from build123d import *

# Parameters (mm, degrees)
SKETCH_1_W          = 31.500863908
SKETCH_1_H          = 82
SKETCH_1_R          = 10.417524335
SKETCH_1_R_2        = 1.56
EXTRUDE_1_DEPTH     = 4
SKETCH_3_W          = 31.500863908
SKETCH_3_H          = 3
EXTRUDE_2_DEPTH     = 35
SKETCH_6_R          = 1.5
CUT_EXTRUDE_1_DEPTH = 4


with BuildPart() as part:
    # 草图1 → 凸台-拉伸1 (new body)
    with BuildSketch(Plane.XY):
        with Locations((0, 14.377078694)):
            Rectangle(SKETCH_1_W, SKETCH_1_H)
        with Locations((0, -6.708333333)):
            Circle(SKETCH_1_R, mode=Mode.SUBTRACT)
        with Locations((0, -20.208333333)):
            Circle(SKETCH_1_R_2, mode=Mode.SUBTRACT)
        with BuildLine():
            Line((8.85, 15.791666667), (-8.85, 15.791666667))
            ThreePointArc((-8.85, 15.791666667), (-10.35, 14.291666667), (-8.85, 12.791666667))
            Line((-8.85, 12.791666667), (8.85, 12.791666667))
            ThreePointArc((8.85, 12.791666667), (10.35, 14.291666667), (8.85, 15.791666667))
        make_face(mode=Mode.SUBTRACT)
    extrude(amount=EXTRUDE_1_DEPTH)

    # 草图3 → 凸台-拉伸2 (add)
    with BuildSketch(Plane(origin=(0, 0, 0), x_dir=(-1, 0, 0), z_dir=(0, 0, -1))):
        with Locations((0, 53.877078694)):
            Rectangle(SKETCH_3_W, SKETCH_3_H)
    extrude(amount=EXTRUDE_2_DEPTH)

    # 草图6 → 切除-拉伸1 (cut, through all)
    with BuildSketch(Plane.XZ.offset(-52.377078694)):
        with Locations((-8.166436246, -9.151254402)):
            Circle(SKETCH_6_R)
        with Locations((8.166436246, -9.151254402)):
            Circle(SKETCH_6_R)
        with Locations((8.166436246, -25.848745598)):
            Circle(SKETCH_6_R)
        with Locations((-8.166436246, -25.848745598)):
            Circle(SKETCH_6_R)
    extrude(amount=-CUT_EXTRUDE_1_DEPTH, mode=Mode.SUBTRACT)


solid = part.part
The model under review builds one solid part; all positions refer to its coordinate system, in mm. A direction names the side the tool comes from. Coordinates: 2 decimals unless noted, no trailing zeros. Write each loop counter-clockwise with the first axis right and the second up, starting at its lowest first coordinate (ties: lowest second). Pieces come first, ordered by that corner, then holes. Notation, with made-up numbers: (-10, 58.5) - (-2, 58.5) arc R36 ccw to (-2, 93.5) - close; hole circle Ø9 at (35.25, 71). An arc over 180 degrees is marked (long way). Answer as CSV lines item,"result".
(1) We need section D-D (x = 12). Give the boundary of the cut face in (y, z).
Data:
outline,"(-26.62, 0) - (52.38, 0) - (52.38, -35) - (55.38, -35) - (55.38, 4) - (-26.62, 4) - close"
(2) Tool access review of faces 1 (the flat face through (0, 52.377, -17)), 2 (the cylindrical face through (10.35, 14.26, 1.97)), 3 (the flat face through (-15.75, 20.3, 0.5)): name each direction out of +Z, -Z, +X, -X, +Y, -Y from which nothing blocks a thin tool from reaching the whole face with its end or side.
Data:
face 1,"-Z, +X, -X, -Y"
face 2,"+Z, -Z"
face 3,"+Z, -Z, -X, +Y, -Y"
(3) We need section C-C (z = 1). Give the boundary of the cut face in (x, y).
Data:
outline,"(-15.75, -26.62) - (15.75, -26.62) - (15.75, 55.38) - (-15.75, 55.38) - close; hole circle Ø20.84 at (0, -6.71); hole (-8.85, 12.79) - (8.85, 12.79) arc R1.5 ccw to (8.85, 15.79) - (-8.85, 15.79) arc R1.5 ccw to start; hole circle Ø3.12 at (0, -20.21)"
(4) Clearance check with flat-ended pins moving along their axes: pin 1 Ø16 at (x, z) = (0.5, -11.5) entering from -Y; pin 2 Ø5 at (x, y) = (0, -20.21) entering from +Z. State where each tip first meets the part, or that it passes through.
Data:
pin 1,"stops at y = 52.38"
pin 2,"stops at z = 4"
(5) For line 1 along Y through (x, z) = (0, 1.8); line 2 along Z through (x, y) = (-9.5, 44); line 3 along Y through (x, z) = (-1, -1), list the stretches that pass through material, from the lowest coordinate up. Write a range as [from, to].
Data:
line 1,"y = [-26.62, -21.77], [-18.65, -17.13], [3.71, 12.79], [15.79, 55.38]"
line 2,"z = [0, 4]"
line 3,"y = [52.38, 55.38]"
(6) We need section A-A (x = 0). Give the boundary of the cut face in (y, z), plus the area to 3 significant figures.
Data:
outline,"(-26.62, 0) - (-21.77, 0) - (-21.77, 4) - (-26.62, 4) - close; (-18.65, 0) - (-17.13, 0) - (-17.13, 4) - (-18.65, 4) - close; (3.71, 0) - (12.79, 0) - (12.79, 4) - (3.71, 4) - close; (15.79, 0) - (52.38, 0) - (52.38, -35) - (55.38, -35) - (55.38, 4) - (15.79, 4) - close"
area,"325 mm2"
(7) Mouldability with a two-part tool opening along Z and no side actions: class faces 4 (the cylindrical face through (6.976, 53.856, -10.064)), 5 (the flat face through (15.75, 20.3, 0.5)), 6 (the flat face through (0, 24, 4)) as pulls with the +Z half, pulls with the -Z half, needs draft (parallel to the pull), parting line crosses it, or undercut.
Data:
face 4,"undercut"
face 5,"needs draft"
face 6,"pulls with the +Z half"
(8) We need section B-B (y = -2). Give the boundary of the cut face in (x, z), plus the area to 3 significant figures.
Data:
outline,"(-15.75, 0) - (-9.29, 0) - (-9.29, 4) - (-15.75, 4) - close; (9.29, 0) - (15.75, 0) - (15.75, 4) - (9.29, 4) - close"
area,"51.7 mm2"
